Geometry check sheet. Reference: the model listing, model coordinates, mm. Face numbers are marked on the shaded views. Round coordinates to 2 decimals unless told otherwise and drop trailing zeros. Loops run counter-clockwise (first coordinate to the right, second up) from the corner with the lowest first, then second, coordinate; pieces in that order, holes last. Notation, with made-up numbers: M -6,51.5 L 36,51.5 A31 ccw 36,78.5 Z; hole C 20.5,-9.75 d3. An arc over 180 degrees is marked long. Write item = value, one per line.
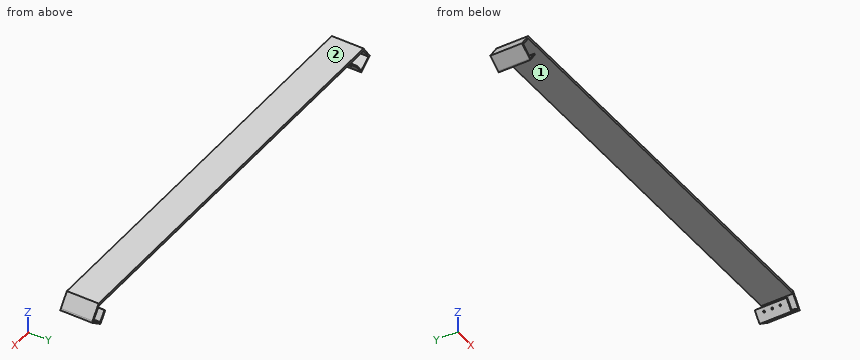
from build123d import *

# Parameters (mm, degrees)
F0_W     = 771.5
F0_H     = 5
F1_DEPTH = 29.5
F2_R     = 1.65
F3_DEPTH = 3
F4_R     = 1.65
F5_DEPTH = 25


with BuildPart() as f1:
    # F0 (on Front) → F1 (new body, symmetric)
    with BuildSketch(Plane.XZ):
        Rectangle(F0_W, F0_H)
        Polygon((403.2728842886, -20.5855475021), (385.75, 2.5), (385.75, -2.5), (400.8649778716, -22.4132479506), align=None)
        Polygon((-385.75, -2.5), (-385.75, 2.5), (-402.2831578173, -21.4661766194), (-399.9460936263, -23.0784092134), align=None)
        Polygon((405.0866816331, -22.9751372562), (403.2728842886, -20.5855475021), (400.8649778716, -22.4132479506), (380.951729921, -37.5282258222), (382.7655272655, -39.9178155762), align=None)
        Polygon((-399.9460936263, -23.0784092134), (-402.2831578173, -21.4661766194), (-403.9866890525, -23.935585725), (-381.0712156481, -39.7439119453), (-379.367684413, -37.2745028397), align=None)
        Polygon((382.7655272655, -39.9178155762), (380.951729921, -37.5282258222), (368.8597476237, -21.5976274617), (366.4701578696, -23.4114248063), (380.3759375115, -41.7316129208), align=None)
        Polygon((-368.0108095119, -20.811775469), (-379.367684413, -37.2745028397), (-381.0712156481, -39.7439119453), (-379.367684413, -40.9190994274), (-366.3072782767, -21.9869629511), align=None)
    extrude(amount=F1_DEPTH, both=True)

    # F2 (on face) → F3 (cut)
    with BuildSketch(Plane(origin=(-237.9157828305, 0, 164.1271049294), x_dir=(0, 1, 0), z_dir=(0.8231363685, 0, -0.5678437451))):
        with Locations((-15, -233.6035655756)):
            Circle(F2_R)
        with Locations((0, -233.6035655756)):
            Circle(F2_R)
        with Locations((15, -233.6035655756)):
            Circle(F2_R)
    extrude(amount=-F3_DEPTH, mode=Mode.SUBTRACT)

    # F4 (on face) → F5 (cut)
    with BuildSketch(Plane(origin=(221.236119488, 0, 167.9273546307), x_dir=(0, -1, 0), z_dir=(-0.796529918, 0, -0.6045991149))):
        with Locations((0, -247.7154333532)):
            Circle(F4_R)
        with Locations((-15, -247.7154333532)):
            Circle(F4_R)
        with Locations((15, -247.7154333532)):
            Circle(F4_R)
    extrude(amount=-F5_DEPTH, mode=Mode.SUBTRACT)


solid = f1.part
(1) Release check for a two-part mould opening along X. For the marked faces 1 and 2 record: released by +X, released by -X, zero draft, split by the parting line, or undercut.
Result set:
face_1 = undercut
face_2 = zero draft
(2) Material ranges on line 1 along X through (y, z) = (-3.5, -23); line 2 along X through (y, z) = (-20, -30); line 3 along Z through (x, y) = (101.5, -12.5), recorded low to high. Write a range as from..to.
Result set:
line_1 = -403.34..-399.89, -369.52..-367.01, 367.01..369.92, 400.09..405.05
line_2 = -395.2..-389.91, -374.35..-371.84, 371.47..375.24, 390.87..395.83
line_3 = -2.5..2.5
(3) Sectioned sample at A-A on x = 215.5. Record the cut outline in (y, z).
Result set:
outline = M -29.5,-2.5 L 29.5,-2.5 L 29.5,2.5 L -29.5,2.5 Z
(4) Depth check by flat-ended pin: pin 1 Ø1.5 at (y, z) = (13, -26.5) entering from -X; pin 2 Ø2 at (y, z) = (-23, -21.5) entering from +X; pin 3 Ø10 at (x, y) = (-250, 20.5) entering from -Z. Enter the tip coordinate at first touch or a pass-through.
Result set:
pin_1 = -401.36
pin_2 = 404.73
pin_3 = -2.5
